Source: CAD feature listing. Evaluate the final solid. Frame: model axes, mm. A direction names the side the tool comes from. Coordinates: 2 decimals unless noted, no trailing zeros. Loops run counter-clockwise (first coordinate to the right, second up) from the corner with the lowest first, then second, coordinate; pieces in that order, holes last.
Item 1: Section query B-B, the plane z = 0. Return the cut outline in (x, y), then the cut area to 3 significant figures.
Item 2: Pull-direction query (Y, two-part tool) for faces 4 (the flat face through (105, 10, 3)), 5 (the flat face through (-56, 870, -56)), 6 (the flat face through (56, 515, 56)), 7 (the flat face through (-25, 20, -85)); classes: +Y half, -Y half, draft (parallel to the pull), parting line (faces both ways), or undercut.
Item 3: Reachability of faces 1 (the flat face through (-81, 8.8, 161)), 2 (the flat face through (56, 870, 56)), 3 (the cylindrical face through (39.22, 480.96, 75.41)) from +Z, -Z, +X, -X, +Y, -Y: full face, straight path, thin tool, end or side. Return the list, or none.
Item 4: Section query D-D, the plane z = 102.5. Return the cut outline in (x, y), then the cut area to 3 significant figures.
Item 5: Section query C-C, the plane y = 331. Return the cut outline in (x, z), then the cut area to 3 significant figures.
Item 6: Line query: probe 1 along Z at (x, y) = (85, 12.25); probe 2 along Z at (x, y) = (-85, 6); probe 3 along Y at (x, z) = (51, -62). Output: solid intervals per line, ascending.
Item 7: Pin query (flat end, axial travel): pin 1 Ø8 at (x, z) = (4.5, -121.5) entering from +Y; pin 2 Ø6 at (x, y) = (-34.5, 729.5) entering from -Z; pin 3 Ø6 at (y, z) = (124.5, 30) entering from -X; pin 4 Ø7 at (x, z) = (-85, -165) entering from +Y. Return the tip coordinate at first contact, or that it passes through.
Item 8: Section query A-A, the plane x = 0. Return the cut outline in (y, z).
```python
from build123d import *

# Parameters (mm, degrees)
SKETCH1_W           = 210
SKETCH1_H           = 370
BOSS_EXTRUDE1_DEPTH = 20
SKETCH2_R           = 85
BOSS_EXTRUDE2_DEPTH = 935
SKETCH3_R           = 75
CUT_EXTRUDE1_DEPTH  = 956
SKETCH4_R           = 4.5
CUT_EXTRUDE2_DEPTH  = 956
SKETCH5_R           = 9
CUT_EXTRUDE3_DEPTH  = 8.8
SKETCH7_W           = 20
SKETCH7_H           = 355
CUT_EXTRUDE4_DEPTH  = 291.060966544
SKETCH8_W           = 20
SKETCH8_H           = 355
CUT_EXTRUDE5_DEPTH  = 291.060966544


with BuildPart() as part:
    # Sketch1 → Boss-Extrude1 (new body)
    with BuildSketch(Plane(origin=(0, 0, 0), x_dir=(1, 0, 0), z_dir=(0, 1, 0))):
        Rectangle(SKETCH1_W, SKETCH1_H)
    extrude(amount=BOSS_EXTRUDE1_DEPTH)

    # Sketch2 → Boss-Extrude2 (add)
    with BuildSketch(Plane(origin=(0, 20, 0), x_dir=(1, 0, 0), z_dir=(0, 1, 0))):
        Circle(SKETCH2_R)
    extrude(amount=BOSS_EXTRUDE2_DEPTH)

    # Sketch3 → Cut-Extrude1 (cut, through all)
    with BuildSketch(Plane(origin=(0, 955, 0), x_dir=(1, 0, 0), z_dir=(0, 1, 0))):
        Circle(SKETCH3_R)
    extrude(amount=-CUT_EXTRUDE1_DEPTH, mode=Mode.SUBTRACT)

    # Sketch4 → Cut-Extrude2 (cut, through all)
    with BuildSketch(Plane.XZ):
        with Locations((-85, 165)):
            Circle(SKETCH4_R)
        with Locations((85, 165)):
            Circle(SKETCH4_R)
        with Locations((85, -165)):
            Circle(SKETCH4_R)
        with Locations((-85, -165)):
            Circle(SKETCH4_R)
    extrude(amount=-CUT_EXTRUDE2_DEPTH, mode=Mode.SUBTRACT)

    # Sketch5 → Cut-Extrude3 (cut)
    with BuildSketch(Plane.XZ):
        with Locations((-85, 165)):
            Circle(SKETCH5_R)
        with Locations((85, 165)):
            Circle(SKETCH5_R)
        with Locations((85, -165)):
            Circle(SKETCH5_R)
        with Locations((-85, -165)):
            Circle(SKETCH5_R)
    extrude(amount=-CUT_EXTRUDE3_DEPTH, mode=Mode.SUBTRACT)

    # Sketch7 → Cut-Extrude4 (cut, through all)
    with BuildSketch(Plane(origin=(60.104076401, 0, 60.104076401), x_dir=(0.707106781, 0, -0.707106781), z_dir=(0.707106781, 0, 0.707106781))):
        with Locations((0, 692.5)):
            Rectangle(SKETCH7_W, SKETCH7_H)
    extrude(amount=-CUT_EXTRUDE4_DEPTH, mode=Mode.SUBTRACT)

    # Sketch8 → Cut-Extrude5 (cut, through all)
    with BuildSketch(Plane(origin=(60.104076401, 0, -60.104076401), x_dir=(-0.707106781, 0, -0.707106781), z_dir=(0.707106781, 0, -0.707106781))):
        with Locations((0, 692.5)):
            Rectangle(SKETCH8_W, SKETCH8_H)
    extrude(amount=-CUT_EXTRUDE5_DEPTH, mode=Mode.SUBTRACT)


solid = part.part
```
Verdict:
1. outline: (-105, 0) - (-75, 0) - (-75, 955) - (-85, 955) - (-85, 20) - (-105, 20) - close; (75, 0) - (105, 0) - (105, 20) - (85, 20) - (85, 955) - (75, 955) - close
1. area: 19,900 mm2
2. face 4: draft
2. face 5: undercut
2. face 6: undercut
2. face 7: +Y half
3. face 1: -Y
3. face 2: none
3. face 3: +Y
4. outline: (-105, 0) - (105, 0) - (105, 20) - (-105, 20) - close
4. area: 4,200 mm2
5. outline: circle Ø170 at (0, 0); hole circle Ø150 at (0, 0)
5. area: 5,030 mm2
6. probe 1: z = -185 to -169.5, -160.5 to 160.5, 169.5 to 185
6. probe 2: z = -185 to -174, -156 to 156, 174 to 185
6. probe 3: y = 0 to 515, 870 to 955
7. pin 1: stops at y = 20
7. pin 2: stops at z = -78.95
7. pin 3: stops at x = -80.6
7. pin 4: passes through
8. outline: (0, -185) - (20, -185) - (20, -85) - (955, -85) - (955, -75) - (0, -75) - close; (0, 75) - (955, 75) - (955, 85) - (20, 85) - (20, 185) - (0, 185) - close
